Geometry check sheet. Reference: the model listing, model coordinates, mm. Coordinates: 2 decimals unless noted, no trailing zeros. Loops run counter-clockwise (first coordinate to the right, second up) from the corner with the lowest first, then second, coordinate; pieces in that order, holes last. Notation, with made-up numbers: (-27.5, 58.25) - (9.5, 58.25) arc R17 cw to (9.5, 87.25) - close; hole circle Ø1 at (69.5, 85.5). An arc over 180 degrees is marked (long way). One line per item, written item: value.
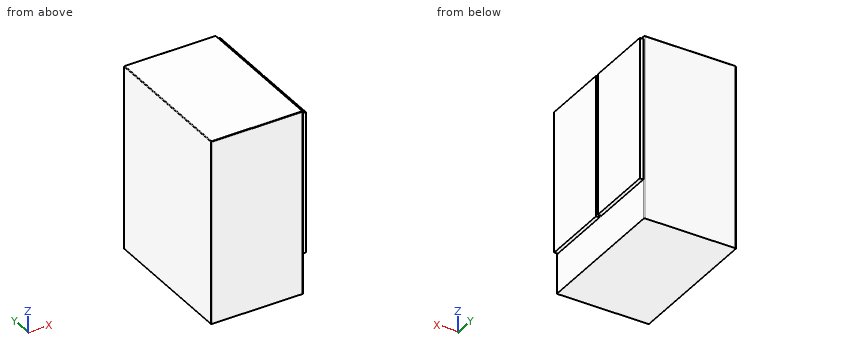
from build123d import *

# Parameters (mm, degrees)
F0_W     = 650
F0_H     = 1300
F1_DEPTH = 1000
F2_W     = 480
F2_H     = 1000
F3_DEPTH = 25
F4_R     = 5


with BuildPart() as f1:
    # F0 (on Front) → F1 (new body)
    with BuildSketch(Plane.XZ):
        with Locations((325, 650)):
            Rectangle(F0_W, F0_H)
    extrude(amount=F1_DEPTH)

    # F2 (on face) → F3 (join)
    with BuildSketch(Plane.YZ.offset(650)):
        with Locations((-250, 780)):
            Rectangle(F2_W, F2_H)
        with Locations((-750, 780)):
            Rectangle(F2_W, F2_H)
    extrude(amount=F3_DEPTH)

    # F4
    f4_edges = [f1.edges().sort_by_distance(p)[0] for p in [
        (325, -1000, 1300),
        (0, -1000, 650),
        (650, -1000, 650),
        (650, -500, 1300),
        (0, -500, 1300),
        (325, 0, 1300),
        (650, 0, 650),
        (0, 0, 650),
    ]]
    fillet(f4_edges, radius=F4_R)


solid = f1.part
(1) Cross-section at A-A on z = 210.5. Record the cut outline in (x, y), and give its area (3 significant figures).
Reply:
outline: (0, -995) arc R5 ccw to (5, -1000) - (645, -1000) arc R5 ccw to (650, -995) - (650, -5) arc R5 ccw to (645, 0) - (5, 0) arc R5 ccw to (0, -5) - close
area: 650,000 mm2
(2) Material ranges on probe 1 along X at (y, z) = (-710.5, 214.5), recorded low to high. Write a range as from..to.
Reply:
probe 1: 0..650
(3) Go/stop test with flat-tipped pins: pin 1 Ø20 at (x, z) = (659, 1024) entering from +Y; pin 2 Ø20 at (x, y) = (666, -751) entering from -Z; pin 3 Ø12.5 at (x, z) = (667, 917.5) entering from -Y. Record where each tip stops, or that it passes through.
Reply:
pin 1: y = -2
pin 2: z = 280
pin 3: y = -990
